Autodesk Fusion 360 part; units mm, degrees
sketch "Sketch1" plane through (0, 0, 0) normal (0, 1, 0) x (1, 0, 0)
  circle A0 centre (0, 0) radius 10
  dimension "d1" = 20
extrude "Extrude1" add sketch "Sketch1" along normal blind 3
fillet "Fillet1" radius 0.5 1 edges at (-9.3233, 3, 3.6162)
fillet "Fillet2" radius 0.5 1 edges at (-9.3233, 0, 3.6162)
sketch "Sketch2" plane through (0, 3, 0) normal (0, 1, 0) x (-1, 0, 0)
  circle A0 centre (0, 0) radius 9.5
  circle A1 centre (0, 0) radius 9.5
  line L0 (2, 7.5) -> (-2, 7.5)
  line L1 (-2, 7.5) -> (-2, -7.5)
  line L2 (-2, -7.5) -> (2, -7.5)
  line L3 (2, -7.5) -> (2, 7.5)
  line L4 (2, 7.5) -> (-2, -7.5) construction
  line L5 (-2, 7.5) -> (2, -7.5) construction
  line L6 (-2, -7.5) -> (-5.5, -7.5)
  line L7 (-5.5, -7.5) -> (-5.5, 7.5)
  line L8 (-5.5, 7.5) -> (-2, 7.5)
  line L9 (-2, 7.5) -> (-2, -7.5)
  line L10 (2, -7.5) -> (5.5, -7.5)
  line L11 (5.5, -7.5) -> (5.5, 7.5)
  line L12 (5.5, 7.5) -> (2, 7.5)
  line L13 (2, 7.5) -> (2, -7.5)
  dimension "d8" = 19
  dimension "d9" = 4
  dimension "d10" = 15
  dimension "d11" = 3.5
  dimension "d12" = 15
  dimension "d13" = 3.5
  dimension "d14" = 15
extrude "Extrude2" add sketch "Sketch2" along normal blind 8 contours L3 L10 L11 L12 L13 | L1 L6 L7 L8 L9
sketch "Sketch3" plane through (5.5, 0, 0) normal (1, 0, 0) x (0, 0, -1)
  line L0 (-7.5, 3) -> (7.5, 3)
  line L1 (7.5, 3) -> (7.5, 11)
  line L2 (7.5, 11) -> (-7.5, 11)
  line L3 (-7.5, 11) -> (-7.5, 3)
  line L4 (0, 3) -> (0, 8) construction
  line L5 (1.5, 9.5) -> (-1.5, 9.5)
  line L6 (-1.5, 9.5) -> (-1.5, 6.5)
  line L7 (-1.5, 6.5) -> (1.5, 6.5)
  line L8 (1.5, 6.5) -> (1.5, 9.5)
  line L9 (1.5, 9.5) -> (-1.5, 6.5) construction
  line L10 (-1.5, 9.5) -> (1.5, 6.5) construction
  point P0 (0, 8)
  dimension "d17" = 5
  dimension "d18" = 3
  dimension "d19" = 3
extrude "Extrude3" cut sketch "Sketch3" against normal blind 16 contours L5 L6 L7 L8
fillet "Fillet3" radius 0.5 16 edges at (5.5, 8, 1.5) (5.5, 9.5, 0) (5.5, 8, -1.5) (5.5, 6.5, 0) (2, 8, 1.5) (2, 9.5, 0) (2, 8, -1.5) (2, 6.5, 0) (-2, 6.5, 0) (-2, 8, 1.5) (-2, 9.5, 0) (-2, 8, -1.5) (-5.5, 8, 1.5) (-5.5, 9.5, 0) (-5.5, 8, -1.5) (-5.5, 6.5, 0)
sketch "Sketch4" plane through (5.5, 0, 0) normal (1, 0, 0) x (0, 0, -1)
  line L0 (-7.5, 3) -> (7.5, 3)
  line L1 (7.5, 3) -> (7.5, 11)
  line L2 (7.5, 11) -> (-7.5, 11)
  line L3 (-7.5, 11) -> (-7.5, 3)
  line L4 (-2, 10) -> (2, 10)
  line L5 (2, 10) -> (2, 6)
  line L6 (2, 6) -> (-2, 6)
  line L7 (-2, 6) -> (-2, 10)
  line L8 (-7.5, 11) -> (-3, 11)
  line L9 (-3, 11) -> (-3, 6)
  line L10 (-3, 6) -> (-7.5, 6)
  line L11 (-7.5, 6) -> (-7.5, 11)
  line L12 (7.5, 11) -> (3, 11)
  line L13 (3, 11) -> (3, 6)
  line L14 (3, 6) -> (7.5, 6)
  line L15 (7.5, 6) -> (7.5, 11)
  dimension "d24" = 4.5
  dimension "d25" = 5
  dimension "d26" = 4.5
  dimension "d27" = 5
extrude "Extrude4" cut sketch "Sketch4" against normal blind 18 contours L2 L3 L8 L9 L10 L11 | L1 L2 L12 L13 L14 L15
sketch "Sketch5" plane through (2, 0, 0) normal (-1, 0, 0) x (0, 0, 1)
  line L0 (-2, 10) -> (2, 10)
  line L1 (2, 10) -> (2, 6)
  line L2 (2, 6) -> (-2, 6)
  line L3 (-2, 6) -> (-2, 10)
  line L4 (7.5, 6) -> (3, 6)
  line L5 (3, 6) -> (3, 11)
  line L6 (3, 11) -> (-3, 11)
  line L7 (-3, 11) -> (-3, 6)
  line L8 (-3, 6) -> (-7.5, 6)
  line L9 (-7.5, 6) -> (-7.5, 3)
  line L10 (-7.5, 3) -> (7.5, 3)
  line L11 (7.5, 3) -> (7.5, 6)
  line L12 (-3, 11) -> (3, 11)
  line L13 (3, 11) -> (3, 10)
  line L14 (3, 10) -> (-3, 10)
  line L15 (-3, 10) -> (-3, 11)
  dimension "d30" = 1
extrude "Extrude5" add sketch "Sketch5" along normal blind 4 contours L0 L5 L6 L7 L12 L13 L14 L15
sketch "Sketch6" plane through (0, 0, 3) normal (0, 0, 1) x (1, 0, 0)
  line L0 (2, 10) -> (2, 6)
  line L1 (2, 6) -> (5.5, 6)
  line L2 (5.5, 6) -> (5.5, 11)
  line L3 (5.5, 11) -> (-5.5, 11)
  line L4 (-5.5, 11) -> (-5.5, 6)
  line L5 (-5.5, 6) -> (-2, 6)
  line L6 (-2, 6) -> (-2, 10)
  line L7 (-2, 10) -> (2, 10)
  line L8 (5.5, 11) -> (5.5, 12.5)
  line L9 (2.5, 15.5) -> (-1.5, 15.5)
  line L10 (-1.5, 15.5) -> (-1.5, 14)
  line L11 (-1.5, 14) -> (2.5, 14)
  line L12 (4, 12.5) -> (4, 11)
  arc A0 (5.5, 12.5) -> (2.5, 15.5) centre (2.5, 12.5) ccw
  arc A1 (4, 12.5) -> (2.5, 14) centre (2.5, 12.5) ccw
  circle A2 centre (-1.5, 14.75) radius 0.75
  point P0 (5.5, 15.5)
  point P1 (4, 14)
  dimension "d33" = 4.5
  dimension "d34" = 7
  dimension "d35" = 1.5
  dimension "d36" = 5.5
  dimension "d37" = 3
  dimension "d38" = 1.5
extrude "Extrude6" add sketch "Sketch6" against normal blind 6 contours L3 L8 L9 L11 L12 A0 A1 A2 | L10 A2 | L10 A2
fillet "Fillet4" radius 0.5 45 edges at (5.5, 9.25, 3) (4.6213, 14.6213, 3) (0.5, 15.5, 3) (-2.25, 14.75, 3) (0.5, 14, 3) (3.5607, 13.5607, 3) (4, 11.75, 3) (-0.75, 11, 3) (-5.5, 8.5, 3) (-2, 8, 3) (0, 10, 3) (2, 8, 3) (2, 6, 5.25) (5.5, 6, 5.25) (-2, 6, 5.25) (-5.5, 6, 5.25) (-3.75, 6, 7.5) (-5.5, 4.5, 7.5) (-2, 4.5, 7.5) (5.5, 4.5, 7.5) (2, 4.5, 7.5) (3.75, 6, 7.5) (4, 11.75, -3) (3.5607, 13.5607, -3) (0.5, 14, -3) (-2.25, 14.75, -3) (0.5, 15.5, -3) (4.6213, 14.6213, -3) (5.5, 9.25, -3) (-0.75, 11, -3) (-5.5, 11, 0) (-5.5, 8.5, -3) (-5.5, 6, -5.25) (-5.5, 4.5, -7.5) (-2, 8, -3) (0, 10, -3) (2, 8, -3) (2, 6, -5.25) (-2, 6, -5.25) (-2, 4.5, -7.5) (2, 4.5, -7.5) (3.75, 6, -7.5) (-3.75, 6, -7.5) (5.5, 6, -5.25) (5.5, 4.5, -7.5)
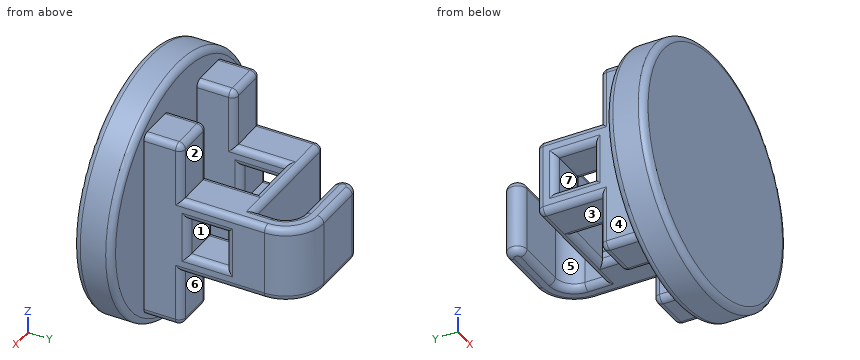
Design review of the part built by this model. Coordinates are the model's own, in mm. Face numbers are marked on the shaded views. A direction names the side the tool comes from. Give positions to 0.01 mm unless a question says otherwise; leave off trailing zeros. Order: outer loops, then holes, each group sorted by start corner. A loop starts at its lowest first (then second) coordinate and runs counter-clockwise, first axis right, second up. Notation, with made-up numbers: M 26.5,18 L 36.5,18 A28 cw 36.5,51 Z; hole C 32.25,78.5 d2. An arc over 180 degrees is marked long. One line per question, with ' | ' between items. Start each with the question number.
Q1. The part is to be moulded in two halves that separate along Y. For the marked faces 1, 2 and 3, say which applies: +Y half, -Y half, draft (parallel to the pull), parting line (faces both ways), or undercut.
Q2. Machinability: for the marked faces 4, 5, 6 and 7, which of the approach directions +Z, -Z, +X, -X, +Y, -Y give a long, thin tool a straight path to every point of the face, cutting with its end or side? Answer none if there is none.
Q3. For pin 1 Ø3.5 at (y, z) = (5, -2.5) entering from +X; pin 2 Ø1.5 at (y, z) = (4, 3.5) entering from -X; pin 3 Ø1.2 at (x, y) = (-4, 7.5) entering from +Z; pin 4 Ø4.5 at (x, z) = (0, 0.5) entering from -Y, all flat-tipped, find the tip position at first contact; note any pin that passes through.
Q4. We need section B-B (y = 3.75). Write out the cut boundary in (x, z).
Q5. We need section C-C (y = 1). Write out the cut boundary in (x, z).
Q6. For L1, parallel to Y at x = -1.25, z = 0; L2, parallel to Z at x = -4.5, y = 8.5; L3, parallel to Y at x = 0.75, z = -6.25, list the stretches that pass through material, from the lowest coordinate up. Write a range as [from, to].
Q7. We need section A-A (x = 0). State how many separate pieces and enclosed holes the cut face has, plus the area to 3 significant figures.
Returned:
1) face 1: undercut | face 2: +Y half | face 3: draft
2) face 4: +Z, -Z, -X, +Y | face 5: +Z, -Z, -X | face 6: -Z, +X, -X, +Y | face 7: +X, -X
3) pin 1: x = 5.5 | pin 2: x = -5.5 | pin 3: z = 3 | pin 4: y = 0
4) outline: M -5.5,-7 A0.5 ccw -5,-7.5 L -2.5,-7.5 A0.5 ccw -2,-7 L -2,7 A0.5 ccw -2.5,7.5 L -5,7.5 A0.5 ccw -5.5,7 Z; M 2,-7 A0.5 ccw 2.5,-7.5 L 5,-7.5 A0.5 ccw 5.5,-7 L 5.5,7 A0.5 ccw 5,7.5 L 2.5,7.5 A0.5 ccw 2,7 Z
5) outline: C 0,0 d20
6) L1: [0, 3], [10, 11], [14, 15.5] | L2: [-3, -1.5], [1.5, 3] | L3: [0, 3]
7) separate pieces: 3 | enclosed holes: 0 | area: 74.4 mm2
